Autodesk Inventor part; units mm, degrees
ref_plane "YZ Plane" through (0, 0, 0) normal (1, 0, 0) x (0, 1, 0)
ref_plane "XZ Plane" through (0, 0, 0) normal (0, 1, 0) x (-1, 0, 0)
ref_plane "XY Plane" through (0, 0, 0) normal (0, 0, 1) x (1, 0, 0)
sketch "Sketch1" plane through (0, 0, 0) normal (0, 0, 1) x (1, 0, 0)
  line L0 (0, 0) -> (164.5, 0)
  line L1 (164.5, 0) -> (164.5, 9)
  line L2 (164.5, 9) -> (0, 9)
  line L3 (0, 9) -> (0, 0)
  circle A0 centre (99, 4) radius 1.6
  circle A1 centre (159.5, 4) radius 1.6
  circle A2 centre (147, 4) radius 1.6
  circle A3 centre (15, 4) radius 1.6
  circle A4 centre (5, 4) radius 1.6
  dimension "d1" = 9
  dimension "d2" = 90
  dimension "d6" = 3.2
  dimension "d7" = 3.2
  dimension "d9" = 60.5
  dimension "d26" = 3.2
  dimension "d27" = 48
  dimension "d28" = 3.2
  dimension "d32" = 15
  dimension "d33" = 5
  dimension "d61" = 3.2
  dimension "d62" = 10
  dimension "d63" = 12.5
  dimension "d108" = 4
  dimension "d109" = 4
  dimension "d111" = 4
  dimension "d112" = 4
  dimension "d113" = 4
ref_plane "Work Plane2" through (0, 0, 0) normal (0, -1, 0) x (1, 0, 0)
sketch "Sketch2" plane through (0, 0, 0) normal (0, -1, 0) x (1, 0, 0)
  circle A0 centre (52, 8) radius 1.6
  circle A1 centre (125, 8) radius 1.6
  circle A2 centre (88.5, 8) radius 1.6
  point P0 (0, 0)
  point P1 (52, 0)
  dimension "d13" = 3.2
  dimension "d15" = 3.2
  dimension "d17" = 3.2
  dimension "d18" = 36.5
  dimension "d64" = 52
  dimension "d65" = 36.5
  dimension "d114" = 8
  dimension "d115" = 73
ref_plane "Work Plane1" through (0, 0, 11) normal (0, 0, 1) x (1, 0, 0)
extrude "klocek" add sketch "Sketch1" along normal blind 11
ref_plane "Work Plane3" through (0, 0, 0) normal (0, -1, 0) x (1, 0, 0)
extrude "prowadzenie osi" cut sketch "Sketch2" against normal up to next
ref_plane "Work Plane4" through (0, 0, 0) normal (0, -1, 0) x (1, 0, 0)
sketch "Sketch7" plane through (0, 0, 0) normal (0, -1, 0) x (1, 0, 0)
  line L0 (0, 11) -> (0, 0)
  line L1 (0, 11) -> (164.5, 11)
  line L2 (0, 11) -> (40, 11)
  line L3 (40, 11) -> (0, 0)
  point P0 (0, -1.8333)
  dimension "d86" = 11
  dimension "d87" = 40
sketch "Sketch8" plane through (0, 0, 0) normal (0, -1, 0) x (1, 0, 0)
  line L0 (164.5, 0) -> (164.5, 11)
  line L1 (164.5, 11) -> (164.5, 3)
  line L2 (164.5, 11) -> (0, 11)
  line L3 (164.5, 11) -> (134.5, 11)
  line L4 (134.5, 11) -> (164.5, 3)
  point P0 (0, 0)
  point P1 (40.8333, 11)
  dimension "d80" = 8
  dimension "d81" = 30
extrude "przedni skos" cut sketch "Sketch7" against normal up to next
extrude "tylni skos" cut sketch "Sketch8" against normal up to next
ref_plane "Work Plane7" through (0, 0, 11) normal (0, 0, 1) x (1, 0, 0)
sketch "Sketch5" plane through (0, 0, 11) normal (0, 0, 1) x (1, 0, 0)
  circle A0 centre (99, 4) radius 1.6
  line L0 (95.5936, 4) -> (97.2968, 6.95)
  line L1 (97.2968, 6.95) -> (100.7032, 6.95)
  line L2 (100.7032, 6.95) -> (102.4064, 4)
  line L3 (102.4064, 4) -> (100.7032, 1.05)
  line L4 (100.7032, 1.05) -> (97.2968, 1.05)
  line L5 (97.2968, 1.05) -> (95.5936, 4)
  point P0 (119.5, 5)
  dimension "d98" = 5.9
extrude "hex insert middle" cut sketch "Sketch5" against normal blind 3
ref_plane "Work Plane6" through (0, 0, 11) normal (0, 0, 1) x (1, 0, 0)
sketch "Sketch9" plane through (0, 0, 11) normal (0, 0, 1) x (1, 0, 0)
  circle A0 centre (147, 4) radius 1.6
  line L0 (150.4064, 4) -> (148.7032, 1.05)
  line L1 (148.7032, 1.05) -> (145.2968, 1.05)
  line L2 (145.2968, 1.05) -> (143.5936, 4)
  line L3 (143.5936, 4) -> (145.2968, 6.95)
  line L4 (145.2968, 6.95) -> (148.7032, 6.95)
  line L5 (148.7032, 6.95) -> (150.4064, 4)
  point P0 (0, 0)
  point P1 (153, 5)
  dimension "d99" = 5.9
extrude "hex insert rear 1" cut sketch "Sketch9" against normal blind 6
ref_plane "Work Plane5" through (0, 0, 11) normal (0, 0, 1) x (1, 0, 0)
sketch "Sketch10" plane through (0, 0, 11) normal (0, 0, 1) x (1, 0, 0)
  circle A0 centre (159.5, 4) radius 1.6
  line L0 (162.9064, 4) -> (161.2032, 1.05)
  line L1 (161.2032, 1.05) -> (157.7968, 1.05)
  line L2 (157.7968, 1.05) -> (156.0936, 4)
  line L3 (156.0936, 4) -> (157.7968, 6.95)
  line L4 (157.7968, 6.95) -> (161.2032, 6.95)
  line L5 (161.2032, 6.95) -> (162.9064, 4)
  point P0 (0, 0)
  dimension "d101" = 5.9
extrude "hex insert rear 2" cut sketch "Sketch10" against normal blind 8.5
sketch "Sketch13" plane through (0, 0, 11) normal (0, 0, 1) x (1, 0, 0)
  line L0 (9.54, 0) -> (-1.59, 0)
  line L1 (7.95, 2.2968) -> (5, 0.5936)
  line L2 (5, 0.5936) -> (2.05, 2.2968)
  line L3 (2.05, 2.2968) -> (2.05, 5.7032)
  line L4 (2.05, 5.7032) -> (5, 7.4064)
  line L5 (5, 7.4064) -> (7.95, 5.7032)
  line L6 (7.95, 5.7032) -> (7.95, 2.2968)
  point P0 (0, 0)
  point P1 (5, 4)
  point P2 (5, 4)
  dimension "d117" = 5.9
extrude "hex insert front 1" cut sketch "Sketch13" against normal through all
sketch "Sketch16" plane through (0, 0, 11) normal (0, 0, 1) x (1, 0, 0)
  circle A0 centre (15, 4) radius 1.6
  line L0 (18.4064, 4) -> (16.7032, 1.05)
  line L1 (16.7032, 1.05) -> (13.2968, 1.05)
  line L2 (13.2968, 1.05) -> (11.5936, 4)
  line L3 (11.5936, 4) -> (13.2968, 6.95)
  line L4 (13.2968, 6.95) -> (16.7032, 6.95)
  line L5 (16.7032, 6.95) -> (18.4064, 4)
  point P0 (0, 0)
  dimension "d93" = 5.9
extrude "hex insert front 2" cut sketch "Sketch16" against normal blind 9
sketch "Sketch17" plane through (0, 0, 0) normal (0, 0, -1) x (-1, 0, 0)
  line L0 (0, 9) -> (0, 0)
  line L1 (0, 0) -> (-5, 0)
  line L2 (-5, 0) -> (-5, 10.0042)
  line L3 (-5, 10.0042) -> (0, 10.0042)
  line L4 (0, 10.0042) -> (0, 0)
  point P0 (-5, 7.4064)
extrude "Extrusion20" cut sketch "Sketch17" against normal up to next
sketch "Sketch18" plane through (40, 0, 11) normal (0, -1, 0) x (1, 0, 0)
  line L0 (9.5, 0) -> (9.5, -2)
  line L1 (9.5, -2) -> (-3.5, -2)
  line L2 (-3.5, -2) -> (-3.5, 0)
  line L3 (-3.5, 0) -> (9.5, 0)
  line L4 (94.5, 0) -> (0, 0)
  circle A0 centre (12, -3) radius 1.6
  line L5 (-35, -11) -> (124.5, -11)
  point P0 (-40, -11)
  dimension "d102" = 2
  dimension "d103" = 13
  dimension "d104" = 2.5
extrude "Extrusion21" cut sketch "Sketch18" against normal blind 7 contours L0 L1 L2 L3
properties part number "wheel_support_v3_narrow_with_line_sensor"
CAD build for the part. Positions are in the model's coordinates, mm. A direction names the side the tool comes from. Round coordinates to 2 decimals unless told otherwise and drop trailing zeros. Order: outer loops, then holes, each group sorted by start corner. A loop starts at its lowest first (then second) coordinate and runs counter-clockwise, first axis right, second up. Notation, with made-up numbers: (27.25, 7) - (79.25, 7) arc R20 ccw to (79.25, 28) - close; hole circle Ø7 at (-10.75, 0). An arc over 180 degrees is marked (long way). Use CSV: the item, a comma, the result in double quotes. Start each with the question number.
1) Saw through at B-B (x = 99). List the corners of the cut face in (y, z).
2) Wall check: L1, parallel to Z at x = 125, y = 2.5; L2, parallel to Y at x = 147, z = 2.5; L3, parallel to X at y = 4.5, z = 1.75. Give the ranges that are in metal, low to high. Write a range as [from, to].
3) Saw through at A-A (x = 125). List the corners of the cut face in (y, z).
4) Two-plate mould, pull along Y, no slides. Class faces 1 (the flat face through (84, 0, 5)), 2 (the cylindrical face through (160.98, 4.61, 1.23)), 3 (the flat face through (43, 3, 9)): pulls with the +Y half, pulls with the -Y half, needs draft (parallel to the pull), parting line crosses it, or undercut.
5) Saw through at C-C (x = 159.5). List the corners of the cut face in (y, z).
6) Tool access for faces 4 (the flat face through (147, 1.05, 6)), 5 (the cylindrical face through (148.48, 4.61, 2.46)): list every direction of +Z, -Z, +X, -X, +Y, -Y with a clear straight run to the whole face (end or side of a thin tool).
7) Pin check, flat tips, straight feed: pin 1 Ø2 at (y, z) = (5, 3) entering from -X; pin 2 Ø1 at (y, z) = (6, 2) entering from -X; pin 3 Ø1.8 at (x, y) = (15.5, 3) entering from +Z. Stop position of each tip, or through.
Values follow:
1,outline,"(0, 0) - (2.4, 0) - (2.4, 8) - (1.05, 8) - (1.05, 11) - (0, 11) - close; (5.6, 0) - (9, 0) - (9, 11) - (6.95, 11) - (6.95, 8) - (5.6, 8) - close"
2,L1,"z = [0, 6.4], [9.6, 11]"
2,L2,"y = [0, 2.4], [5.6, 9]"
2,L3,"x = [7.95, 13.48], [16.52, 97.48], [100.52, 145.48], [148.52, 157.98], [161.02, 164.5]"
3,outline,"(0, 0) - (9, 0) - (9, 6.4) - (0, 6.4) - close; (0, 9.6) - (9, 9.6) - (9, 11) - (0, 11) - close"
4,face 1,"pulls with the -Y half"
4,face 2,"undercut"
4,face 3,"needs draft"
5,outline,"(0, 0) - (2.4, 0) - (2.4, 2.5) - (1.05, 2.5) - (1.05, 4.33) - (0, 4.33) - close; (5.6, 0) - (9, 0) - (9, 4.33) - (6.95, 4.33) - (6.95, 2.5) - (5.6, 2.5) - close"
6,face 4,"+Z"
6,face 5,"+Z, -Z"
7,pin 1,"stops at x = 7.95"
7,pin 2,"stops at x = 6.63"
7,pin 3,"stops at z = 2"
